Source: CAD feature listing. Evaluate the final solid. Frame: model axes, mm. A direction names the side the tool comes from. Give positions to 0.01 mm unless a question says otherwise; leave off trailing zeros. Write each loop counter-clockwise with the first axis right and the second up, starting at its lowest first coordinate (ties: lowest second). Pieces come first, ordered by that corner, then holes. Notation, with made-up numbers: M 30.25,44 L 59.25,44 A28 ccw 59.25,62 Z; hole C 26,22.25 d2. An arc over 180 degrees is marked long. Use CSV: the item, a comma, the result in double quotes. Start each with the question number.
Autodesk Inventor part; units mm, degrees
ref_plane "YZ Plane" through (0, 0, 0) normal (1, 0, 0) x (0, 1, 0)
ref_plane "XZ Plane" through (0, 0, 0) normal (0, 1, 0) x (-1, 0, 0)
ref_plane "XY Plane" through (0, 0, 0) normal (0, 0, 1) x (1, 0, 0)
sketch "Sketch1" plane through (0, 0, 0) normal (0, 1, 0) x (-1, 0, 0)
  line L0 (0, 0) -> (23, 0)
  line L1 (23, 0) -> (23, -23)
  line L2 (23, -23) -> (0, -23)
  line L3 (0, -23) -> (0, 0)
  dimension "d0" = 23
  dimension "d1" = 23
extrude "Extrusion1" add sketch "Sketch1" along normal blind 23
sketch "Sketch2" plane through (0, 23, 0) normal (0, 1, 0) x (1, 0, 0)
  circle A0 centre (-11.5, 11.5) radius 1.5
  line L0 (0, 0) -> (0, 23)
  line L1 (-23, 0) -> (0, 0)
  circle A1 centre (-11.5, 11.5) radius 3
  dimension "d4" = 3
  dimension "d5" = 11.5
  dimension "d6" = 11.5
  dimension "d7" = 6
extrude "Extrusion2" cut sketch "Sketch2" against normal blind 1
sketch "Sketch3" plane through (-23, 0, 0) normal (0, 0, 1) x (1, 0, 0)
  line L0 (6, 16) -> (19, 16)
  line L1 (17, 12) -> (6, 12)
  line L2 (0, 0) -> (0, 23)
  line L3 (23, 0) -> (23, 23)
  line L4 (0, 23) -> (23, 23)
  arc A0 (6, 16) -> (6, 12) centre (6, 14) ccw
  arc A1 (17, 12) -> (17, 16) centre (17, 14) ccw
  point P0 (4, 14)
  dimension "d13" = 7
  dimension "d16" = 4
  dimension "d17" = 6
  dimension "d18" = 6
extrude "Extrusion3" add sketch "Sketch3" along normal blind 1
fillet "Fillet1" radius 1 12 edges at (-11.5, 23, 0) (0, 11.5, 0) (0, 23, -11.5) (-23, 23, -11.5) (-11.5, 23, -23) (-23, 11.5, 0) (0, 11.5, -23) (0, 0, -11.5) (-11.5, 0, 0) (-11.5, 0, -23) (-23, 11.5, -23) (-23, 0, -11.5)
properties part number "Runcam"
1. Section C-C on y = 8.25. Return loops of the section in (x, z), then the cut area to 3 significant figures.
2. First-contact query: pin 1 (1 mm diameter, centred on x = -9.5, y = 19.5, fed in from +Z); pin 2 (0.8 mm diameter, centred on x = -12, z = 0.5, fed in from +Y); pin 3 (0.8 mm diameter, centred on x = -9.5, z = 0.5, fed in from -Y). Flat tips, straight axial feed; report the tip coordinate or a pass-through.
3. Access query for faces 5 (the flat face through (-10, 22, -10)), 6 (the flat face through (-11.6, 16, 0.5)), 7 (the flat face through (-11.4, 12, 0.5)). Directions: +Z, -Z, +X, -X, +Y, -Y. A direction counts if a zero-diameter tool reaches every point of the face in a straight line with its end or side. Return the directions, or none.
4. Section A-A on x = -7.25. Return loops of the section in (y, z), then the cut area to 3 significant figures.
5. Section B-B on y = 14. Return loops of the section in (x, z).
6. Section D-D on x = -11.5. Return loops of the section in (y, z), then the cut area to 3 significant figures.
7. Pull-direction query (X, two-part tool) for faces 1 (the flat face through (0, 11, -12)), 2 (the cylindrical face through (-11.353, 0.285, -22.699)), 3 (the cylindrical face through (-13, 22.51, -11.57)), 4 (the cylindrical face through (-13.9, 22.5, -9.7)); classes: released by +X, released by -X, zero draft, split by the parting line, or undercut.
8. Line query: probe 1 along Z at (x, y) = (-11.5, 22.25); probe 2 along Z at (x, y) = (-11.5, 22.4). Output: solid intervals per line, ascending.
Resolved:
1,outline,"M -23,-22 A1 ccw -22,-23 L -1,-23 A1 ccw 0,-22 L 0,-1 A1 ccw -1,0 L -22,0 A1 ccw -23,-1 Z"
1,area,"528 mm2"
2,pin 1,"stops at z = 0"
2,pin 2,"stops at y = 16"
2,pin 3,"stops at y = 12"
3,face 5,"+Y"
3,face 6,"+Z, +X, -X, +Y"
3,face 7,"+Z, +X, -X, -Y"
4,outline,"M 0,-22 A1 ccw 1,-23 L 22,-23 A1 ccw 23,-22 L 23,-1 A1 ccw 22,0 L 16,0 L 16,1 L 12,1 L 12,0 L 1,0 A1 ccw 0,-1 Z"
4,area,"532 mm2"
5,outline,"M -23,-22 A1 ccw -22,-23 L -1,-23 A1 ccw 0,-22 L 0,-1 A1 ccw -1,0 L -4,0 L -4,1 L -19,1 L -19,0 L -22,0 A1 ccw -23,-1 Z"
6,outline,"M 0,-22 A1 ccw 1,-23 L 22,-23 A1 ccw 23,-22 L 23,-14.5 L 22,-14.5 L 22,-13 L 23,-13 L 23,-10 L 22,-10 L 22,-8.5 L 23,-8.5 L 23,-1 A1 ccw 22,0 L 16,0 L 16,1 L 12,1 L 12,0 L 1,0 A1 ccw 0,-1 Z"
6,area,"529 mm2"
7,face 1,"released by +X"
7,face 2,"zero draft"
7,face 3,"undercut"
7,face 4,"undercut"
8,probe 1,"z = -22.97 to -14.5, -13 to -10, -8.5 to -0.03"
8,probe 2,"z = -22.92 to -14.5, -13 to -10, -8.5 to -0.08"
